Verification items for this drawing (mm, ordinates from the low corner). Round coordinates to 2 decimals unless told otherwise and drop trailing zeros. Loops run counter-clockwise (first coordinate to the right, second up) from the corner with the lowest first, then second, coordinate; pieces in that order, holes last. Notation, with made-up numbers: (-10, -0.5) -> (24, -0.5) arc R22 cw to (24, 23.5) -> close; hole circle Ø5 at (84.5, 56). An arc over 180 degrees is marked (long way). Use a Markdown table: item, result. Add a question column.
Q1. Gauge pin test, flat ends, axial feed: P1, Ø1.5, axis at y = 5, z = 62.5, coming from the -X side (1 decimal); P2, Ø4, axis at y = 5.5, z = 68, coming from the +X side; P3, Ø2, axis at x = 134, y = 7, coming from the -Z side (1 decimal). Record the tip position at first contact, or that the pin passes through.
Q2. Sectioned sample at D-D, the plane y = 4.5. Enter the section's corners in (x, z), then the cut area to 3 significant figures.
Q3. Sectioned sample at A-A, the plane z = 100. Enter the section's corners in (x, y), then the cut area to 4 significant figures.
Q4. Material ranges on L1, parallel to Y at x = 150.5, z = 98; L2, parallel to X at y = 3.25, z = 20; L3, parallel to Z at x = 185, y = 4 (1 decimal), recorded low to high.
Q5. Release check for a two-part mould opening along X. For the marked faces 1, 2 and 3 record: released by +X, released by -X, zero draft, split by the parting line, or undercut.
Q6. Sectioned sample at C-C, the plane x = 23.5. Enter the section's corners in (y, z), then the cut area to 3 significant figures.
Q7. Sectioned sample at B-B, the plane z = 178.5. Enter the section's corners in (x, y).
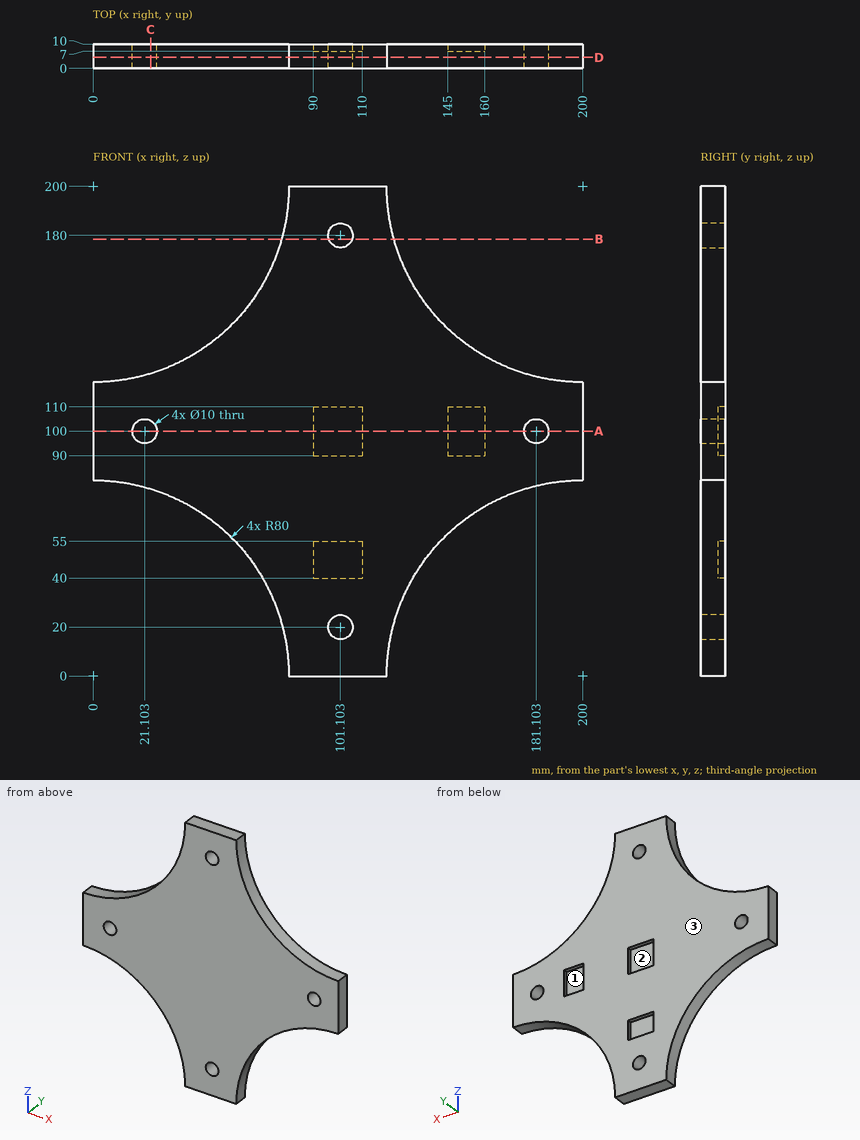
Values:
| question | item | result |
|---|---|---|
| 1 | P1 | x = 49 |
| 1 | P2 | x = 161.27 |
| 1 | P3 | z = 43.7 |
| 2 | outline | (0, 80) arc R80 cw to (80, 0) -> (120, 0) arc R80 cw to (200, 80) -> (200, 120) arc R80 cw to (120, 200) -> (80, 200) arc R80 cw to (0, 120) -> close; hole circle Ø10 at (21.1, 100); hole circle Ø10 at (101.1, 20); hole circle Ø10 at (101.1, 180); hole circle Ø10 at (181.1, 100) |
| 2 | area | 19,600 mm^2 |
| 3 | outline | (0, 0) -> (16.1, 0) -> (16.1, 10) -> (0, 10) -> close; (26.1, 0) -> (176.1, 0) -> (176.1, 10) -> (160, 10) -> (160, 7) -> (145, 7) -> (145, 10) -> (110, 10) -> (110, 7) -> (90, 7) -> (90, 10) -> (26.1, 10) -> close; (186.1, 0) -> (200, 0) -> (200, 10) -> (186.1, 10) -> close |
| 3 | area | 1,695 mm^2 |
| 4 | L1 | 0 to 7 |
| 4 | L2 | 77.46 to 96.1, 106.1 to 122.54 |
| 4 | L3 | 78.6 to 96.9, 103.1 to 121.4 |
| 5 | face 1 | undercut |
| 5 | face 2 | undercut |
| 5 | face 3 | zero draft |
| 6 | outline | (0, 76.47) -> (10, 76.47) -> (10, 95.61) -> (0, 95.61) -> close; (0, 104.39) -> (10, 104.39) -> (10, 123.53) -> (0, 123.53) -> close |
| 6 | area | 383 mm^2 |
| 7 | outline | (77.06, 0) -> (96.33, 0) -> (96.33, 10) -> (77.06, 10) -> close; (105.87, 0) -> (122.94, 0) -> (122.94, 10) -> (105.87, 10) -> close |
